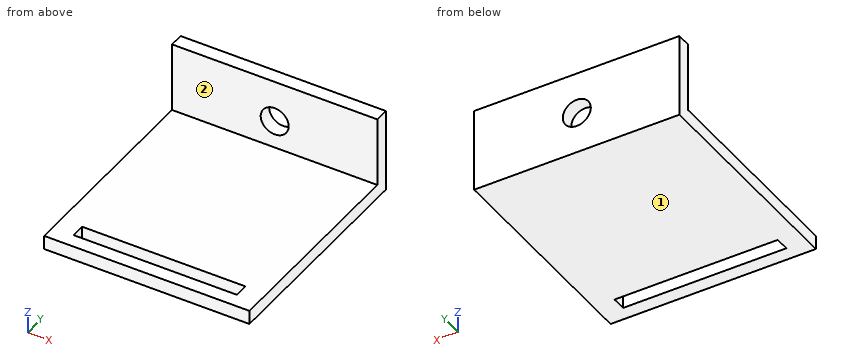
from build123d import *

# Parameters (mm, degrees)
ESTRUSIONE_ESTRUSIONE6_DEPTH = 44
SCHIZZO9_W                   = 35
SCHIZZO9_H                   = 3
TAGLIO_ESTRUSIONE2_DEPTH     = 44
SCHIZZO10_R                  = 3
TAGLIO_ESTRUSIONE3_DEPTH     = 10


with BuildPart() as part:
    # Schizzo8 → Estrusione-Estrusione6 (new body)
    with BuildSketch(Plane(origin=(0, 0, 0), x_dir=(0, 0, -1), z_dir=(1, 0, 0))):
        Polygon((0, 0), (0, 3), (18, 3), (18, -45), (15, -45), (15, 0), align=None)
    extrude(amount=ESTRUSIONE_ESTRUSIONE6_DEPTH)

    # Schizzo9 → Taglio-Estrusione2 (cut)
    with BuildSketch(Plane.XY.offset(-15)):
        with Locations((22, -40.5)):
            Rectangle(SCHIZZO9_W, SCHIZZO9_H)
    extrude(amount=-TAGLIO_ESTRUSIONE2_DEPTH, mode=Mode.SUBTRACT)

    # Schizzo10 → Taglio-Estrusione3 (cut)
    with BuildSketch(Plane(origin=(0, 3, 0), x_dir=(1, 0, 0), z_dir=(0, 1, 0))):
        with Locations((22, 9)):
            Circle(SCHIZZO10_R)
    extrude(amount=-TAGLIO_ESTRUSIONE3_DEPTH, mode=Mode.SUBTRACT)


solid = part.part
Design review of the part built by this model. Coordinates are the model's own, in mm. Face numbers are marked on the shaded views. A direction names the side the tool comes from. Round coordinates to 2 decimals unless told otherwise and drop trailing zeros. Write each loop counter-clockwise with the first axis right and the second up, starting at its lowest first coordinate (ties: lowest second). Pieces come first, ordered by that corner, then holes.
Item 1: Consider section D-D on y = -15. Give the boundary of the cut face in (x, z), and give its area (3 significant figures).
Item 2: For the marked faces 1 and 2, list the 3-axis set-ups (+Z, -Z, +X, -X, +Y, -Y) from which the entire face can be reached by the end or side of a thin tool; tool diameter is ignored.
Item 3: Consider section B-B on x = 30. Give the boundary of the cut face in (y, z).
Item 4: Consider section A-A on x = 22. Give the boundary of the cut face in (y, z).
Item 5: For pin 1 Ø5 at (x, z) = (10, -4.5) entering from -Y; pin 2 Ø5 at (x, y) = (16, -26) entering from +Z, all flat-tipped, find the tip position at first contact; note any pin that passes through.
Item 6: Wall thickness on L1, parallel to X at y = 1.9, z = -9; L2, parallel to Z at x = 22, y = 0.8; L3, parallel to Z at x = 3.5, y = -36.5: over which ranges is each line inside the solid? List them lowest first.
Item 7: Consider section C-C on z = -9. Give the boundary of the cut face in (x, y).
Check values:
1. outline: (0, -18) - (44, -18) - (44, -15) - (0, -15) - close
1. area: 132 mm2
2. face 1: -Z, +X, -X, +Y, -Y
2. face 2: +Z, +X, -X, -Y
3. outline: (-45, -18) - (-42, -18) - (-42, -15) - (-45, -15) - close; (-39, -18) - (3, -18) - (3, 0) - (0, 0) - (0, -15) - (-39, -15) - close
4. outline: (-45, -18) - (-42, -18) - (-42, -15) - (-45, -15) - close; (-39, -18) - (3, -18) - (3, -12) - (0, -12) - (0, -15) - (-39, -15) - close; (0, -6) - (3, -6) - (3, 0) - (0, 0) - close
5. pin 1: stops at y = 0
5. pin 2: stops at z = -15
6. L1: x = 0 to 19, 25 to 44
6. L2: z = -18 to -12, -6 to 0
6. L3: z = -18 to -15
7. outline: (0, 0) - (19, 0) - (19, 3) - (0, 3) - close; (25, 0) - (44, 0) - (44, 3) - (25, 3) - close
